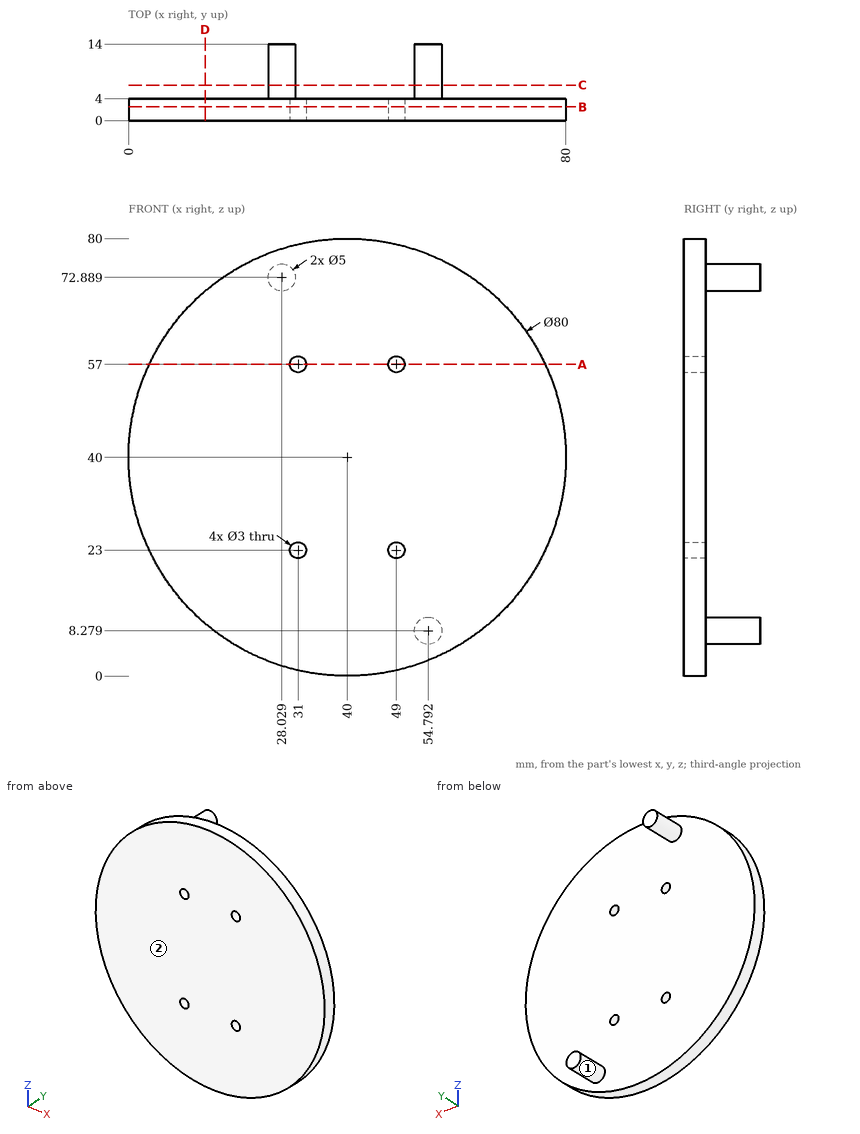
Source: three-view drawing plus pictorial views. Frame: mm from the lowest corner of the part. A direction names the side the tool comes from. Give positions to 0.01 mm unless a question says otherwise; leave off trailing zeros. Write each loop counter-clockwise with the first axis right and the second up, starting at its lowest first coordinate (ties: lowest second). Pieces come first, ordered by that corner, then holes.
(1) Cut plane D-D, the plane x = 14. Return loops of the section in (y, z), then the cut area to 3 significant figures.
(2) Cut plane C-C, the plane y = 6.5. Return loops of the section in (x, z).
(3) Cut plane B-B, the plane y = 2.5. Return loops of the section in (x, z), then the cut area to 3 significant figures.
(4) Cut plane A-A, the plane z = 57. Return loops of the section in (x, y), then the cut area to 3 significant figures.
(5) First-contact query: P1, Ø1.5, axis at x = 56, y = 6.5, coming from the +Z side; P2, Ø5, axis at x = 37.5, y = 7, coming from the +Z side; P3, Ø3, axis at y = 1.5, z = 30, coming from the +X side; P4, Ø6, axis at x = 41.5, z = 8, coming from the +Y side. Flat tips, straight axial feed; report the tip coordinate or a pass-through.
(6) Access query for the marked faces 1 and 2. Directions: +Z, -Z, +X, -X, +Y, -Y. A direction counts if a zero-diameter tool reaches every point of the face in a straight line with its end or side. Return the directions, or none.
(7) Ray query, line 1 (X direction, y = 1.8, z = 23); line 2 (Y direction, x = 35.5, z = 39); line 3 (Z direction, x = 28, y = 6.5). Return the intervals inside material, ascending.
Values follow:
1. outline: (0, 9.6) - (4, 9.6) - (4, 70.4) - (0, 70.4) - close
1. area: 243 mm2
2. outline: circle Ø5 at (28.03, 72.89); circle Ø5 at (54.79, 8.28)
3. outline: circle Ø80 at (40, 40); hole circle Ø3 at (31, 23); hole circle Ø3 at (31, 57); hole circle Ø3 at (49, 23); hole circle Ø3 at (49, 57)
3. area: 5,000 mm2
4. outline: (3.79, 0) - (29.5, 0) - (29.5, 4) - (3.79, 4) - close; (32.5, 0) - (47.5, 0) - (47.5, 4) - (32.5, 4) - close; (50.5, 0) - (76.21, 0) - (76.21, 4) - (50.5, 4) - close
4. area: 266 mm2
5. P1: stops at z = 10.74
5. P2: passes through
5. P3: stops at x = 79.09
5. P4: stops at y = 4
6. face 1: +Y
6. face 2: +Z, -Z, +X, -X, -Y
7. line 1: x = 3.79 to 29.5, 32.5 to 47.5, 50.5 to 76.21
7. line 2: y = 0 to 4
7. line 3: z = 70.39 to 75.39
